Geometry: final body of the model. Coordinates: model frame, mm. Face numbers are marked on the shaded views. A direction names the side the tool comes from. Coordinates: 2 decimals unless noted, no trailing zeros. Loops run counter-clockwise (first coordinate to the right, second up) from the corner with the lowest first, then second, coordinate; pieces in that order, holes last. Notation, with made-up numbers: (81, 38) - (96, 38) arc R10 ccw to (96, 54) - close; hole circle Ø9 at (-14, 47.5). An arc over 180 degrees is marked (long way). Write each question's results on one line, items separated by ' | '. Start each with the question number.
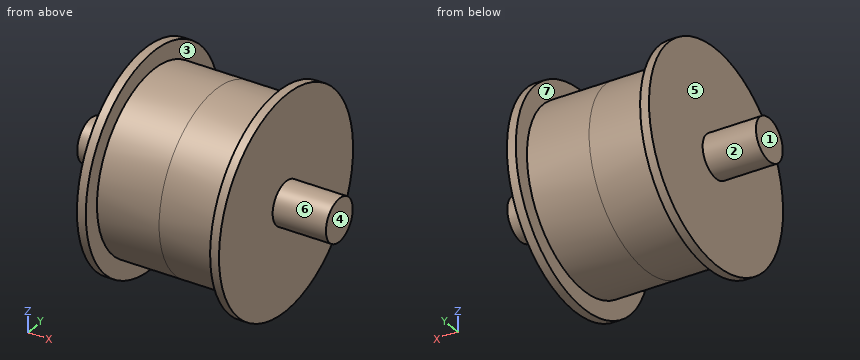
from build123d import *

# Parameters (mm, degrees)
SKETCH3_R           = 6
BOSS_EXTRUDE1_DEPTH = 15
SKETCH4_R           = 30
BOSS_EXTRUDE2_DEPTH = 2.5
BOSS_EXTRUDE3_START = 2.5
SKETCH4_3_R         = 25
BOSS_EXTRUDE3_DEPTH = 17.5


with BuildPart() as part:
    # Sketch3 → Boss-Extrude1 (new body)
    with BuildSketch(Plane(origin=(0, 0, 0), x_dir=(0, 0, -1), z_dir=(1, 0, 0))):
        Circle(SKETCH3_R)
    boss_extrude1 = extrude(amount=-BOSS_EXTRUDE1_DEPTH)

    # Sketch4 → Boss-Extrude2 (add)
    with BuildSketch(Plane(origin=(0, 0, 0), x_dir=(0, 0, -1), z_dir=(1, 0, 0))):
        Circle(SKETCH4_R)
    boss_extrude2 = extrude(amount=BOSS_EXTRUDE2_DEPTH)

    # Sketch4<3> → Boss-Extrude3 (add)
    with BuildSketch(Plane(origin=(0, 0, 0), x_dir=(0, 0, -1), z_dir=(1, 0, 0)).offset(BOSS_EXTRUDE3_START)):
        Circle(SKETCH4_3_R)
    boss_extrude3 = extrude(amount=BOSS_EXTRUDE3_DEPTH)

    # Mirror1: Boss-Extrude3 across plane
    add(boss_extrude3.mirror(Plane(origin=(20, 0, 0), x_dir=(0, 0, 1), z_dir=(1, 0, 0))))

    # Mirror2: Boss-Extrude2 across plane
    add(boss_extrude2.mirror(Plane(origin=(20, 0, 0), x_dir=(0, 0, 1), z_dir=(1, 0, 0))))

    # Mirror3: Boss-Extrude1 across plane
    add(boss_extrude1.mirror(Plane(origin=(20, 0, 0), x_dir=(0, 0, 1), z_dir=(1, 0, 0))))


solid = part.part
1) Material intervals for line 1 (X direction, y = -20.5, z = 15.5); line 2 (X direction, y = 18.5, z = -3); line 3 (Y direction, x = -3.5, z = 0), sorted ascending. Write a range as [from, to].
2) Pin query (flat end, axial travel): pin 1 Ø4 at (x, z) = (13.5, 22.5) entering from +Y; pin 2 Ø2 at (x, y) = (25.5, 7) entering from -Z; pin 3 Ø2 at (x, z) = (25, -9) entering from +Y. Return the tip coordinate at first contact, or that it passes through.
3) Pull-direction query (X, two-part tool) for the marked faces 4, 5, 6 and 7; classes: released by +X, released by -X, zero draft, split by the parting line, or undercut.
4) Section query A-A on y = -24. Output: boundary loops of the cut face in (x, z), and give its area (3 significant figures).
5) Section query D-D on y = 0. Output: boundary loops of the cut face in (x, z).
6) Section query C-C on x = 32. Output: boundary loops of the cut face in (y, z).
7) Access query for the marked faces 1, 2 and 3. Directions: +Z, -Z, +X, -X, +Y, -Y. A direction counts if a zero-diameter tool reaches every point of the face in a straight line with its end or side. Return the directions, or none.
8) Section query B-B on z = -2. Output: boundary loops of the cut face in (x, y), and give its area (3 significant figures).
Returned:
1) line 1: x = [0, 2.5], [37.5, 40] | line 2: x = [0, 40] | line 3: y = [-6, 6]
2) pin 1: stops at y = 14.31 | pin 2: stops at z = -24.27 | pin 3: stops at y = 23.69
3) face 4: released by +X | face 5: released by -X | face 6: zero draft | face 7: undercut
4) outline: (0, -18) - (2.5, -18) - (2.5, -7) - (37.5, -7) - (37.5, -18) - (40, -18) - (40, 18) - (37.5, 18) - (37.5, 7) - (2.5, 7) - (2.5, 18) - (0, 18) - close | area: 670 mm²
5) outline: (-15, -6) - (0, -6) - (0, -30) - (2.5, -30) - (2.5, -25) - (37.5, -25) - (37.5, -30) - (40, -30) - (40, -6) - (55, -6) - (55, 6) - (40, 6) - (40, 30) - (37.5, 30) - (37.5, 25) - (2.5, 25) - (2.5, 30) - (0, 30) - (0, 6) - (-15, 6) - close
6) outline: circle Ø50 at (0, 0)
7) face 1: +Z, -Z, -X, +Y, -Y | face 2: -X | face 3: none
8) outline: (-15, -5.66) - (0, -5.66) - (0, -29.93) - (2.5, -29.93) - (2.5, -24.92) - (37.5, -24.92) - (37.5, -29.93) - (40, -29.93) - (40, -5.66) - (55, -5.66) - (55, 5.66) - (40, 5.66) - (40, 29.93) - (37.5, 29.93) - (37.5, 24.92) - (2.5, 24.92) - (2.5, 29.93) - (0, 29.93) - (0, 5.66) - (-15, 5.66) - close | area: 2,380 mm²
